from build123d import *

# Parameters (mm, degrees)
SKETCH1_W                      = 49
SKETCH1_H                      = 28.7
BOSS_EXTRUDE1_DEPTH            = 5.5
CBORE_FOR_M3_SHCS1_D           = 3.4
CBORE_FOR_M3_SHCS1_CBORE_D     = 5.75
CBORE_FOR_M3_SHCS1_CBORE_DEPTH = 3.4
CBORE_FOR_M3_SHCS2_D           = 3.4
CBORE_FOR_M3_SHCS2_CBORE_D     = 5.75
CBORE_FOR_M3_SHCS2_CBORE_DEPTH = 3.4
SKETCH9_R                      = 11.75
SKETCH9_R_2                    = 10.25
BOSS_EXTRUDE2_DEPTH            = 2
FILLET1_R                      = 1
CHAMFER1_SIZE                  = 1


with BuildPart() as part:
    # Sketch1 → Boss-Extrude1 (new body)
    with BuildSketch(Plane(origin=(0, 0, 0), x_dir=(1, 0, 0), z_dir=(0, 1, 0))):
        Rectangle(SKETCH1_W, SKETCH1_H)
    extrude(amount=BOSS_EXTRUDE1_DEPTH)

    # CBORE for M3 SHCS1 (through all)
    with Locations(Plane(origin=(0, 5.5, 0), x_dir=(1, 0, 0), z_dir=(0, 1, 0))):
        with Locations((-20, 10.45), (20, 10.45), (20, -10.45), (-20, -10.45)):
            CounterBoreHole(CBORE_FOR_M3_SHCS1_D / 2, CBORE_FOR_M3_SHCS1_CBORE_D / 2, CBORE_FOR_M3_SHCS1_CBORE_DEPTH)

    # CBORE for M3 SHCS2 (through all)
    with Locations(Plane(origin=(0, 0, 0), x_dir=(-1, 0, 0), z_dir=(0, -1, 0))):
        with Locations((-5.480077554, -5.480077554), (5.480077554, -5.480077554), (5.480077554, 5.480077554), (-5.480077554, 5.480077554)):
            CounterBoreHole(CBORE_FOR_M3_SHCS2_D / 2, CBORE_FOR_M3_SHCS2_CBORE_D / 2, CBORE_FOR_M3_SHCS2_CBORE_DEPTH)

    # Sketch9 → Boss-Extrude2 (add)
    with BuildSketch(Plane(origin=(0, 5.5, 0), x_dir=(1, 0, 0), z_dir=(0, 1, 0))):
        with Locations(Location((0, 0, 0), (0, 0, 270))):
            Circle(SKETCH9_R)
        with Locations(Location((0, 0, 0), (0, 0, 270))):
            Circle(SKETCH9_R_2, mode=Mode.SUBTRACT)
    extrude(amount=BOSS_EXTRUDE2_DEPTH)

    # Fillet1
    fillet1_edges = [part.edges().sort_by_distance(p)[0] for p in [
        (0, 5.5, -11.75),
        (0, 7.5, -11.75),
    ]]
    fillet(fillet1_edges, radius=FILLET1_R - 0.0001)  # a hair under: the kernel refuses the full size

    # Chamfer1
    chamfer1_edges = [part.edges().sort_by_distance(p)[0] for p in [
        (24.5, 5.5, 0),
        (0, 5.5, -14.35),
        (-24.5, 5.5, 0),
        (0, 5.5, 14.35),
    ]]
    chamfer(chamfer1_edges, length=CHAMFER1_SIZE)


solid = part.part
Source: CAD feature listing. Evaluate the final solid. Frame: model axes, mm. A direction names the side the tool comes from. Round coordinates to 2 decimals unless told otherwise and drop trailing zeros. Loops run counter-clockwise (first coordinate to the right, second up) from the corner with the lowest first, then second, coordinate; pieces in that order, holes last. Notation, with made-up numbers: M 10.25,75.5 L 23.25,75.5 A21 cw 23.25,98.5 Z; hole C 26,-39 d3. An arc over 180 degrees is marked long. Return JSON: item names as keys, results as strings. Group by question number.
1. Pin query (flat end, axial travel): pin 1 (4.5 mm diameter, centred on x = -5.48, z = -5.48, fed in from +Y); pin 2 (6 mm diameter, centred on x = 19.5, z = 5, fed in from -Y); pin 3 (1.7 mm diameter, centred on x = -21, z = 9.5, fed in from +Y); pin 4 (4 mm diameter, centred on x = 5.48, z = -5.48, fed in from -Y). Return the tip coordinate at first contact, or that it passes through.
2. Reachability of faces 4 (the face through (0, 2, 14.35)), 5 (the face through (-7.03, 1.68, 3.06)), 6 (the face through (0, 5.5, 0)) from +Z, -Z, +X, -X, +Y, -Y: full face, straight path, thin tool, end or side. Return the list, or none.
3. Mould query, pull axis Z, two halves, no side actions, for faces 1 (the face through (-3.86, 4.46, -5.99)), 2 (the face through (-0.34, 4.99, 13.86)), 3 (the face through (-24, 5, 0)). Classes: released by +Z, released by -Z, zero draft, split by the parting line, or undercut.
4. Section query A-A on x = -20. Output: boundary loops of the cut face in (y, z) (3 decimals).
5. Material intervals for line 1 along Z through (x, y) = (-20, 2.95) (3 decimals); line 2 along X through (y, z) = (1.3, -10.45); line 3 along Z through (x, y) = (-20, 1), sorted ascending. Write a range as from..to.
6. Section query C-C on y = 1. State how many separate pieces and enclosed holes the cut face has, and give its area (3 significant figures).
Checks:
{
 "1": {"pin 1": "stops at y = 5.5", "pin 2": "stops at y = 0", "pin 3": "stops at y = 2.1", "pin 4": "stops at y = 3.4"},
 "2": {"face 4": "+Z, +X, -X, +Y, -Y", "face 5": "-Y", "face 6": "+Y"},
 "3": {"face 1": "undercut", "face 2": "released by +Z", "face 3": "zero draft"},
 "4": {"outline": "M 0,-14.35 L 4.5,-14.35 L 5.5,-13.35 L 5.5,-13.325 L 2.1,-13.325 L 2.1,-12.15 L 0,-12.15 Z; M 0,-8.75 L 2.1,-8.75 L 2.1,-7.575 L 5.5,-7.575 L 5.5,7.575 L 2.1,7.575 L 2.1,8.75 L 0,8.75 Z; M 0,12.15 L 2.1,12.15 L 2.1,13.325 L 5.5,13.325 L 5.5,13.35 L 4.5,14.35 L 0,14.35 Z"},
 "5": {"line 1": "z = -14.35..-13.325, -7.575..7.575, 13.325..14.35", "line 2": "x = -24.5..-21.7, -18.3..18.3, 21.7..24.5", "line 3": "z = -14.35..-12.15, -8.75..8.75, 12.15..14.35"},
 "6": {"separate pieces": "1", "enclosed holes": "8", "area": "1,270 mm²"}
}
